Verification items for the finished model (mm, model axes). A direction names the side the tool comes from. Give positions to 0.01 mm unless a question says otherwise; leave off trailing zeros. Write each loop counter-clockwise with the first axis right and the second up, starting at its lowest first coordinate (ties: lowest second). Pieces come first, ordered by that corner, then holes. Notation, with made-up numbers: (88, -4) - (99, -4) arc R24 ccw to (99, 7) - close; hole circle Ø11 at (-34.5, 71). An arc over 180 degrees is marked (long way). Answer as a JSON object with one key per item and string values. Group by question number.
Item 1: Go/stop test with flat-tipped pins: pin 1 (1.5 mm diameter, centred on y = -0.5, z = 0.5, fed in from -X); pin 2 (0.9 mm diameter, centred on x = 6, z = 1.5, fed in from -Y). Record where each tip stops, or that it passes through.
Item 2: Sectioned sample at B-B, the plane z = 1.8. Record the boundary of the cut face in (x, y), and give its area (3 significant figures).
Item 3: Scan lines: line 1 along Y through (x, z) = (-9, 2.8); line 2 along X through (y, z) = (0.5, 1.5); line 3 along X through (y, z) = (7.25, 1.2). Record each from-to range of solid material in increasing order. Write a range as [from, to].
Item 4: Tool access check on faces 1 (the face through (21, -8, 1)), 2 (the face through (79.807, -0.176, 1.479)), 3 (the face through (21, 0, 3.5)), 4 (the face through (-36.19, 0.18, 1.48)), 5 (the face through (23, 8, 1)). Record the directions out of +Z, -Z, +X, -X, +Y, -Y that give a thin tool (end or side, any length) a straight path to the whole face; none if there is none.
Item 5: Sectioned sample at A-A, the plane x = 57. Record the boundary of the cut face in (y, z).
```python
from build123d import *

# Parameters (mm, degrees)
F1_DEPTH    = 3
F3_DEPTH    = 0.5
F4_T1_DEPTH = 100
F4_T4_ANGLE = 180
F4_T6_ANGLE = 180


# Not quite as in the source:
# - a fillet or chamfer that OpenCascade refuses, or shapes differently, is made with other operations: its cross-section is extruded or revolved along the edge and cut away or added


with BuildPart() as f1:
    # F0 (on Top) → F1 (new body)
    with BuildSketch(Plane.XY):
        with BuildLine():
            Line((71.8090593611, 7.9999995343), (-28.1909406389, 7.9999995343))
            ThreePointArc((-28.1909406389, 7.9999995343), (-36.1909406389, -4.657e-07), (-28.1909406389, -8.0000004657))
            Line((-28.1909406389, -8.0000004657), (71.8090593611, -8.0000004657))
            ThreePointArc((71.8090593611, -8.0000004657), (79.8090593611, -4.657e-07), (71.8090593611, 7.9999995343))
        make_face()
    extrude(amount=F1_DEPTH)

    # F2 (on face) → F3 (join)
    with BuildSketch(Plane.XY.offset(3)):
        with BuildLine():
            Line((71.8090593611, 8.9999995343), (-28.1909406389, 8.9999995343))
            ThreePointArc((-28.1909406389, 8.9999995343), (-37.1909406389, -4.657e-07), (-28.1909406389, -9.0000004657))
            Line((-28.1909406389, -9.0000004657), (71.8090593611, -9.0000004657))
            ThreePointArc((71.8090593611, -9.0000004657), (80.8090593611, -4.657e-07), (71.8090593611, 8.9999995343))
        make_face()
        with BuildLine():
            Line((-28.1909406389, 7.9999995343), (71.8090593611, 7.9999995343))
            ThreePointArc((71.8090593611, 7.9999995343), (79.8090593611, -4.657e-07), (71.8090593611, -8.0000004657))
            Line((71.8090593611, -8.0000004657), (-28.1909406389, -8.0000004657))
            ThreePointArc((-28.1909406389, -8.0000004657), (-36.1909406389, -4.657e-07), (-28.1909406389, 7.9999995343))
        make_face(mode=Mode.SUBTRACT)
        with BuildLine():
            ThreePointArc((71.8090593611, -8.0000004657), (79.8090593611, -4.657e-07), (71.8090593611, 7.9999995343))
            Line((71.8090593611, 7.9999995343), (-28.1909406389, 7.9999995343))
            ThreePointArc((-28.1909406389, 7.9999995343), (-36.1909406389, -4.657e-07), (-28.1909406389, -8.0000004657))
            Line((-28.1909406389, -8.0000004657), (71.8090593611, -8.0000004657))
        make_face()
    extrude(amount=F3_DEPTH)

    # F4: fillet of radius 5 on 4 edges, made by hand

    # F4_s2 → F4_t1 (cut)
    with BuildSketch(Plane.YZ.offset(-28.1909406389)):
        with BuildLine():
            ThreePointArc((-9.0000004657, 3), (-7.9385849826, 3.3733971724), (-6.8205509939, 3.5))
            Line((-6.8205509939, 3.5), (-9.0000004657, 3.5))
            Line((-9.0000004657, 3.5), (-9.0000004657, 3))
        make_face()
        with BuildLine():
            ThreePointArc((8.9999995343, 3), (7.9385840513, 3.3733971724), (6.8205500626, 3.5))
            Line((6.8205500626, 3.5), (8.9999995343, 3.5))
            Line((8.9999995343, 3.5), (8.9999995343, 3))
        make_face()
    extrude(amount=F4_T1_DEPTH, mode=Mode.SUBTRACT)

    # F4_s3 → F4_t4 (revolve, cut)
    with BuildSketch(Plane.YZ.offset(-28.1909406389)):
        with BuildLine():
            ThreePointArc((8.9999995343, 3), (7.9385840513, 3.3733971724), (6.8205500626, 3.5))
            Line((6.8205500626, 3.5), (8.9999995343, 3.5))
            Line((8.9999995343, 3.5), (8.9999995343, 3))
        make_face()
    revolve(axis=Axis((-28.1909406389, -4.657e-07, 3.5), (0, 0, 1)), revolution_arc=F4_T4_ANGLE, mode=Mode.SUBTRACT)

    # F4_s5 → F4_t6 (revolve, cut)
    with BuildSketch(Plane.YZ.offset(71.8090593611)):
        with BuildLine():
            ThreePointArc((-6.8205509939, 3.5), (-7.9385849826, 3.3733971724), (-9.0000004657, 3))
            Line((-9.0000004657, 3), (-9.0000004657, 3.5))
            Line((-9.0000004657, 3.5), (-6.8205509939, 3.5))
        make_face()
    revolve(axis=Axis((71.8090593611, -4.657e-07, 3.5), (0, 0, 1)), revolution_arc=F4_T6_ANGLE, mode=Mode.SUBTRACT)


solid = f1.part
```
Geometry check:
{
 "1": {"pin 1": "x = -36.19", "pin 2": "y = -8"},
 "2": {"outline": "(-28.19, -8) - (71.81, -8) arc R8 ccw to (71.81, 8) - (-28.19, 8) arc R8 ccw to start", "area": "1,800 mm^2"},
 "3": {"line 1": "[-8, 8]", "line 2": "[-36.18, 79.79]", "line 3": "[-31.57, 75.19]"},
 "4": {"face 1": "-Z, +X, -X, -Y", "face 2": "-Z, +X", "face 3": "+Z, +X, -X, +Y, -Y", "face 4": "-Z, -X", "face 5": "-Z, +X, -X, +Y"},
 "5": {"outline": "(-9, 3) - (-8, 3) - (-8, 0) - (8, 0) - (8, 3) - (9, 3) arc R5 ccw to (6.82, 3.5) - (-6.82, 3.5) arc R5 ccw to start"}
}
